```python
from build123d import *

# Parameters (mm, degrees)
F1_DEPTH = 17


with BuildPart() as f1:
    # F0 (on Top) → F1 (new body)
    with BuildSketch(Plane.XY):
        with BuildLine():
            Line((-18.694246, 28.693632), (-18.694246, 30.693632))
            Line((-18.694246, 30.693632), (-31.694246, 30.693632))
            ThreePointArc((-31.694246, 30.693632), (-34.522673, 29.522059), (-35.694246, 26.693632))
            Line((-35.694246, 26.693632), (-35.694246, 24.693632))
            Line((-35.694246, 24.693632), (-33.694246, 24.693632))
            ThreePointArc((-33.694246, 24.693632), (-32.522673, 27.522059), (-29.694246, 28.693632))
            Line((-29.694246, 28.693632), (-18.694246, 28.693632))
        make_face()
    extrude(amount=F1_DEPTH)


solid = f1.part
```
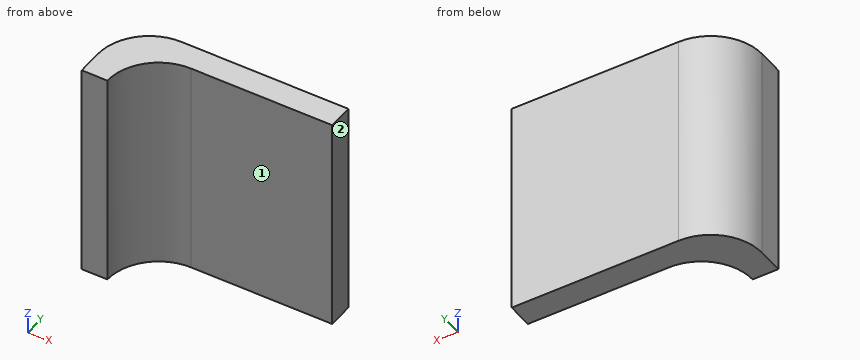
Input: part model. Units: mm. Frame: model coordinates. Face numbers are marked on the shaded views. A direction names the side the tool comes from. Coordinates: 2 decimals unless noted, no trailing zeros. Order: outer loops, then holes, each group sorted by start corner. A loop starts at its lowest first (then second) coordinate and runs counter-clockwise, first axis right, second up. Notation, with made-up numbers: (-2.75, -10.75) - (10.25, -10.75) arc R22 ccw to (10.25, 25.25) - close; hole circle Ø5 at (-18.75, 24.5). An arc over 180 degrees is marked (long way). Return JSON: item names as keys, results as strings.
Q1. Ray query, probe 1 along Y at (x, z) = (-22.75, 15.5); probe 2 along X at (y, z) = (26.75, 13.5); probe 3 along X at (y, z) = (29.5, 3.25). Return the intervals inside material, ascending.
The answers:
{"probe 1": "y = 28.69 to 30.69", "probe 2": "x = -35.69 to -33.13", "probe 3": "x = -34.54 to -18.69"}
Q2. Cut plane B-B (x = -22). Return loops of the section in (y, z), then the cut area to 3 significant figures.
The answers:
{"outline": "(28.69, 0) - (30.69, 0) - (30.69, 17) - (28.69, 17) - close", "area": "34.0 mm2"}
Q3. Cut plane A-A (z = 2). Return loops of the section in (x, y).
The answers:
{"outline": "(-35.69, 24.69) - (-33.69, 24.69) arc R4 cw to (-29.69, 28.69) - (-18.69, 28.69) - (-18.69, 30.69) - (-31.69, 30.69) arc R4 ccw to (-35.69, 26.69) - close"}
Q4. Cut plane C-C (y = 30). Return loops of the section in (x, z), then the cut area to 3 significant figures.
The answers:
{"outline": "(-33.95, 0) - (-18.69, 0) - (-18.69, 17) - (-33.95, 17) - close", "area": "259 mm2"}
Q5. Access query for the marked faces 1 and 2. Directions: +Z, -Z, +X, -X, +Y, -Y. A direction counts if a zero-diameter tool reaches every point of the face in a straight line with its end or side. Return the directions, or none.
The answers:
{"face 1": "+Z, -Z, +X, -Y", "face 2": "+Z, -Z, +X, +Y, -Y"}
Q6. First-contact query: pin 1 (3 mm diameter, centred on x = -27, y = 27, fed in from -Z); pin 2 (9 mm diameter, centred on x = -23.5, z = 11.5, fed in from -Y). Flat tips, straight axial feed; report the tip coordinate or a pass-through.
The answers:
{"pin 1": "passes through", "pin 2": "stops at y = 28.69"}
